from build123d import *

# Parameters (mm, degrees)
F0_R     = 38.1
F1_DEPTH = 76.2
F3_DEPTH = 76.201
F4_R     = 6.35


with BuildPart() as f1:
    # F0 (on Top) → F1 (new body)
    with BuildSketch(Plane.XY):
        Circle(F0_R)
    extrude(amount=F1_DEPTH)

    # F2 (on face) → F3 (cut, through all)
    with BuildSketch(Plane.XY.offset(76.2)):
        Polygon((0.456082, 22.861894), (-21.602016, 7.498473), (-13.806862, -18.227582), (13.068906, -18.763739), (21.88389, 6.630954), align=None)
    extrude(amount=-F3_DEPTH, mode=Mode.SUBTRACT)

    # F4
    f4_edges = [f1.edges().sort_by_distance(p)[0] for p in [
        (-38.1, 0, 76.2),
    ]]
    fillet(f4_edges, radius=F4_R)


solid = f1.part
For this review, take the finished solid that the model builds, in its own axes (mm). A direction names the side the tool comes from. Round coordinates to 2 decimals unless told otherwise and drop trailing zeros. Order: outer loops, then holes, each group sorted by start corner. A loop starts at its lowest first (then second) coordinate and runs counter-clockwise, first axis right, second up. Notation, with made-up numbers: M 9.5,-32 L 52.5,-32 A11 cw 52.5,-19 Z; hole C 80,-7 d2. An arc over 180 degrees is marked long. Write each question's results on one line, items separated by ' | '. Start each with the question number.
1. To check wall thickness, follow L1, parallel to X at y = -7, z = 30.5; L2, parallel to X at y = 2.5, z = 11.5; L3, parallel to Y at x = 0.5, z = 51. State the ranges of each line that lie inside material, in increasing order. Write a range as [from, to].
2. Add section B-B (y = 0). State the section outline as (x, z) points.
3. Tool access review of faces 4 (the face through (0, -21, 76.2)), 5 (the face through (17.415, -6.244, 38.633)): name each direction out of +Z, -Z, +X, -X, +Y, -Y from which nothing blocks a thin tool from reaching the whole face with its end or side.
4. Clearance check with flat-ended pins moving along their axes: pin 1 Ø6 at (x, z) = (6.5, 28.5) entering from -Y; pin 2 Ø4 at (y, z) = (22.5, 59.5) entering from +X; pin 3 Ø12 at (x, z) = (-19, 16.5) entering from +Y. State where each tip first meets the part, or that it passes through.
5. Draft analysis for pull direction X (two halves, no side actions). For faces 1 (the face through (7.9, 17.5, 0)), 2 (the face through (-30.235, -23.183, 34.436)), 3 (the face through (-17.76, -5.18, 38.63)), state which applies: pulls with the +X half, pulls with the -X half, needs draft (parallel to the pull), parting line crosses it, or undercut.
6. Add section A-A (z = 64.5). State the section outline as (x, y) points, then the cut area to 3 significant figures.
Output values:
1) L1: [-37.45, -17.21], [17.15, 37.45] | L2: [-38.02, -20.09], [20.45, 38.02] | L3: [-38.1, -18.51], [22.83, 38.1]
2) outline: M -38.1,0 L -19.33,0 L -19.33,76.2 L -31.75,76.2 A6.35 ccw -38.1,69.85 Z; M 19.58,0 L 38.1,0 L 38.1,69.85 A6.35 ccw 31.75,76.2 L 19.58,76.2 Z
3) face 4: +Z, +X, -X, +Y, -Y | face 5: +Z, -Z
4) pin 1: y = -37.94 | pin 2: x = 32.11 | pin 3: y = 35.81
5) face 1: needs draft | face 2: parting line crosses it | face 3: undercut
6) outline: C 0,0 d76.2; hole M -21.6,7.5 L -13.81,-18.23 L 13.07,-18.76 L 21.88,6.63 L 0.46,22.86 Z | area: 3,320 mm^2
